Here's how the part is built. I have some questions about the finished solid (model axes, mm). A direction names the side the tool comes from. Coordinates: 2 decimals unless noted, no trailing zeros. Write each loop counter-clockwise with the first axis right and the second up, starting at its lowest first coordinate (ties: lowest second). Pieces come first, ordered by that corner, then holes. Notation, with made-up numbers: (31, 8.25) -> (39, 8.25) arc R21 ccw to (39, 35.25) -> close; hole circle Ø5 at (46.5, 77). An arc over 180 degrees is marked (long way). Use a Markdown table: item, result. Add a question column.
```python
from build123d import *

# Parameters (mm, degrees)
SKETCH1_R               = 3
BOSS_EXTRUDE1_DEPTH     = 6
CUT_EXTRUDE1_DEPTH      = 15.696938457
CUT_EXTRUDE1_DEPTH_BACK = 15.696938457
SKETCH2_W               = 14
SKETCH2_H               = 6
SKETCH3_R               = 5
SKETCH3_R_2             = 2.5
BOSS_EXTRUDE2_DEPTH     = 12
FILLET1_R               = 1


with BuildPart() as part:
    # Sketch1 → Boss-Extrude1 (new, symmetric)
    with BuildSketch(Plane.XY):
        with BuildLine():
            Line((0, -6), (12, -6))
            Line((12, -6), (12, 6))
            Line((12, 6), (0, 6))
            ThreePointArc((0, 6), (-6, 0), (0, -6))
        make_face()
        Circle(SKETCH1_R, mode=Mode.SUBTRACT)
    extrude(amount=BOSS_EXTRUDE1_DEPTH, both=True)

    # Sketch2 → Cut-Extrude1 (cut, two sides: drawn at the far end of the back side and taken through both)
    with BuildSketch(Plane(origin=(0, 0, 0), x_dir=(1, 0, 0), z_dir=(0, 1, 0)).offset(-CUT_EXTRUDE1_DEPTH_BACK)):
        with Locations((1, 0)):
            Rectangle(SKETCH2_W, SKETCH2_H)
    extrude(amount=CUT_EXTRUDE1_DEPTH + CUT_EXTRUDE1_DEPTH_BACK, mode=Mode.SUBTRACT)

    # Sketch3 → Boss-Extrude2 (add)
    with BuildSketch(Plane(origin=(12, 0, 0), x_dir=(0, 0, -1), z_dir=(1, 0, 0))):
        with Locations(Location((0, 0, 0), (0, 0, 180))):
            Circle(SKETCH3_R)
        Circle(SKETCH3_R_2, mode=Mode.SUBTRACT)
    extrude(amount=BOSS_EXTRUDE2_DEPTH)

    # Fillet1
    fillet1_edges = [part.edges().sort_by_distance(p)[0] for p in [
        (12, 0, -5),
    ]]
    fillet(fillet1_edges, radius=FILLET1_R - 0.0001)  # a hair under: the kernel refuses the full size


solid = part.part
```
Q1. Please list where these lines run through material, in increasing order: line 1 (Y direction, x = 0, z = 5.4); line 2 (Y direction, x = 16, z = 0); line 3 (X direction, y = 0, z = -4.95).
Q2. Thinking about a two-plate mould opening in X: for faces 1 (the flat face through (12, -4, 5)), 2 (the cylindrical face through (-3, 0, 4)), 3 (the cylindrical face through (18, 0, -5)), which applies, released by +X, released by -X, zero draft, split by the parting line, or undercut?
Q3. Suppose I cut it at D-D, the plane x = 17.25. Write out the boundary of the cut face in (y, z), and give its area (3 significant figures).
Q4. Suppose I cut it at A-A, the plane y = 0. State how many separate pieces and enclosed holes the cut face has, and give its area (3 significant figures).
Q5. Suppose I cut it at B-B, the plane x = -2. Write out the boundary of the cut face in (y, z).
Q6. Which directions (+Z, -Z, +X, -X, +Y, -Y) give clear straight access to the entire face, cutting with the end or side of a thin tool? Please do faces 4 (the flat face through (24, 2, 2)), 5 (the flat face through (12, 0, 0)), 6 (the flat face through (8, 0, 0)).
Q7. Will these pins go through, and if not, where does the flat tip stop? pin 1 (3 mm diameter, centred on y = 2.5, z = -0.5, fed in from -X); pin 2 (4 mm diameter, centred on x = 19, y = -3.5, fed in from +Z); pin 3 (2 mm diameter, centred on x = 15, z = 1, fed in from -Y).
Answer key:
| question | item | result |
|---|---|---|
| 1 | line 1 | y = -6 to -3, 3 to 6 |
| 1 | line 2 | y = -5 to -2.5, 2.5 to 5 |
| 1 | line 3 | x = -6 to -3, 3 to 24 |
| 2 | face 1 | released by +X |
| 2 | face 2 | undercut |
| 2 | face 3 | zero draft |
| 3 | outline | circle Ø10 at (0, 0); hole circle Ø5 at (0, 0) |
| 3 | area | 58.9 mm^2 |
| 4 | separate pieces | 3 |
| 4 | enclosed holes | 0 |
| 4 | area | 156 mm^2 |
| 5 | outline | (-5.66, -6) -> (-2.24, -6) -> (-2.24, -3) -> (-5.66, -3) -> close; (-5.66, 3) -> (-2.24, 3) -> (-2.24, 6) -> (-5.66, 6) -> close; (2.24, -6) -> (5.66, -6) -> (5.66, -3) -> (2.24, -3) -> close; (2.24, 3) -> (5.66, 3) -> (5.66, 6) -> (2.24, 6) -> close |
| 6 | face 4 | +Z, -Z, +X, +Y, -Y |
| 6 | face 5 | +X |
| 6 | face 6 | -X, +Y, -Y |
| 7 | pin 1 | stops at x = 8 |
| 7 | pin 2 | stops at z = 4.77 |
| 7 | pin 3 | stops at y = -5 |
